from build123d import *

# Parameters (mm, degrees)
F1_DEPTH = 50.8


with BuildPart() as f1:
    # F0 (on Front) → F1 (new body)
    with BuildSketch(Plane.XZ):
        with BuildLine():
            Line((-86.453595, 4.343704), (-60.966483, -48.488677))
            Line((-60.966483, -48.488677), (-2.468743, -52.832381))
            Line((-2.468743, -52.832381), (30.541885, -4.343704))
            Line((30.541885, -4.343704), (5.054773, 48.488677))
            Line((5.054773, 48.488677), (-53.442967, 52.832381))
            ThreePointArc((-53.442967, 52.832381), (-83.945756, 38.11739), (-86.453595, 4.343704))
        make_face()
    extrude(amount=-F1_DEPTH)


solid = f1.part
For this review, take the finished solid that the model builds, in its own axes (mm). Coordinates: 2 decimals unless noted, no trailing zeros. Order: outer loops, then holes, each group sorted by start corner. A loop starts at its lowest first (then second) coordinate and runs counter-clockwise, first axis right, second up. Notation, with made-up numbers: (12.5, 78.25) - (40.5, 78.25) arc R15 cw to (40.5, 83.25) - close; hole circle Ø9 at (-28.75, 15). An arc over 180 degrees is marked (long way). Answer as CSV lines item,"result". Start each with the question number.
1) Add section C-C (x = -65.5). State the section outline as (y, z) points.
2) Add section B-B (z = 25.5). State the section outline as (x, y) points, then the cut area to 3 significant figures.
3) Insertion check: P1, Ø3, axis at y = 5.5, z = -7.5, coming from the -X side; P2, Ø4, axis at x = -17.5, y = 40.5, coming from the -Z side; P3, Ø1.5, axis at x = 13.5, z = 34, coming from the -Y side; P4, Ø5, axis at y = 32, z = 1.5, coming from the +X side. Each pin has a flat end and moves straight along its axis. Give the tip position at first contact, or say it passes through.
4) To check wall thickness, follow line 1 along Z through (x, y) = (-52.5, 14); line 2 along Z through (x, y) = (-70, 7.5); line 3 along X through (y, z) = (42.5, 43.5). State the ranges of each line that lie inside material, in increasing order. Write a range as [from, to].
5) Add section A-A (y = 12.5). State the section outline as (x, z) points, then the cut area to 3 significant figures.
Result:
1,outline,"(0, -39.09) - (50.8, -39.09) - (50.8, 51.55) - (0, 51.55) - close"
2,outline,"(-89.2, 0) - (16.14, 0) - (16.14, 50.8) - (-89.2, 50.8) - close"
2,area,"5,350 mm^2"
3,P1,"x = -81.46"
3,P2,"z = -51.86"
3,P3,"through"
3,P4,"x = 28.93"
4,line 1,"[-49.12, 52.76]"
4,line 2,"[-29.76, 49.87]"
4,line 3,"[-79.39, 7.46]"
5,outline,"(-86.45, 4.34) - (-60.97, -48.49) - (-2.47, -52.83) - (30.54, -4.34) - (5.05, 48.49) - (-53.44, 52.83) arc R33.87 ccw to start"
5,area,"9,640 mm^2"
